Source: CAD feature listing. Evaluate the final solid. Frame: model axes, mm. Give positions to 0.01 mm unless a question says otherwise; leave off trailing zeros. Order: outer loops, then holes, each group sorted by start corner. A loop starts at its lowest first (then second) coordinate and runs counter-clockwise, first axis right, second up. Notation, with made-up numbers: M 42,-14.5 L 80,-14.5 A34 cw 80,20.5 Z; hole C 89,84 d4. An arc over 180 degrees is marked long. Answer as a JSON object with one key per item and string values. Group by question number.
1. Material intervals for L1, parallel to X at y = -1.25, z = -10.5; L2, parallel to Y at x = 2.5, z = 15.5; L3, parallel to Y at x = 2, z = -6, sorted ascending. Write a range as [from, to].
2. Section query A-A (z = -12.5). Output: boundary loops of the cut face in (x, y) (3 decimals), plus the area to 3 significant figures.
3. Pin query (flat end, axial travel): P1, Ø1, axis at x = 1, z = 4, coming from the +Y side; P2, Ø2, axis at x = -1.5, z = 12.5, coming from the -Y side. Return the tip coordinate at first contact, or that it passes through.
from build123d import *

# Parameters (mm, degrees)
SKETCH1_R           = 3.175
BOSS_EXTRUDE1_DEPTH = 20.6375
CUT_EXTRUDE1_START  = -0.127
SKETCH6_R           = 3.175
SKETCH6_R_2         = 3.048
CUT_EXTRUDE1_DEPTH  = 0.127
CUT_EXTRUDE2_START  = -0.127
SKETCH7_R           = 3.175
SKETCH7_R_2         = 3.048
CUT_EXTRUDE2_DEPTH  = 0.127
FILLET1_R           = 0.254


with BuildPart() as part:
    # Sketch1 → Boss-Extrude1 (new, symmetric)
    with BuildSketch(Plane.XY):
        Circle(SKETCH1_R)
    extrude(amount=BOSS_EXTRUDE1_DEPTH, both=True)

    # Sketch6 → Cut-Extrude1 (cut)
    with BuildSketch(Plane(origin=(0, 0, -4.8895), x_dir=(-1, 0, 0), z_dir=(0, 0, -1)).offset(CUT_EXTRUDE1_START)):
        Circle(SKETCH6_R)
        Circle(SKETCH6_R_2, mode=Mode.SUBTRACT)
    extrude(amount=CUT_EXTRUDE1_DEPTH, mode=Mode.SUBTRACT)

    # Sketch7 → Cut-Extrude2 (cut)
    with BuildSketch(Plane(origin=(0, 0, 4.7625), x_dir=(-1, 0, 0), z_dir=(0, 0, -1)).offset(CUT_EXTRUDE2_START)):
        Circle(SKETCH7_R)
        Circle(SKETCH7_R_2, mode=Mode.SUBTRACT)
    extrude(amount=CUT_EXTRUDE2_DEPTH, mode=Mode.SUBTRACT)

    # Fillet1
    fillet1_edges = [part.edges().sort_by_distance(p)[0] for p in [
        (-3.175, 0, -20.6375),
        (-3.175, 0, 20.6375),
    ]]
    fillet(fillet1_edges, radius=FILLET1_R)


solid = part.part
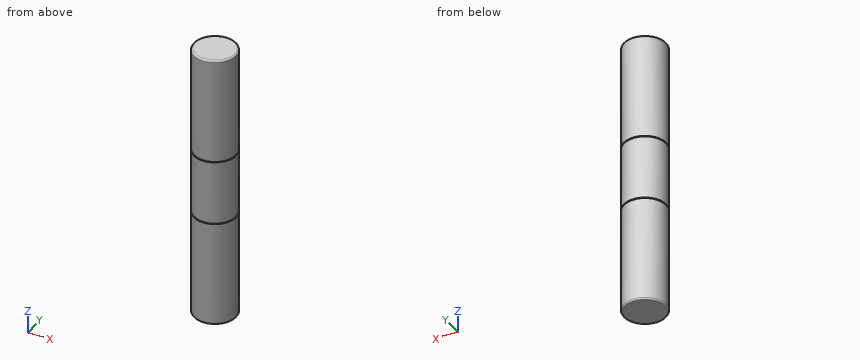
Answer sheet:
{
 "1": {"L1": "[-2.92, 2.92]", "L2": "[-1.96, 1.96]", "L3": "[-2.47, 2.47]"},
 "2": {"outline": "C 0,0 d6.35", "area": "31.7 mm^2"},
 "3": {"P1": "y = 3.14", "P2": "y = -3.14"}
}
